```python
from build123d import *

# Parameters (mm, degrees)
FACE001_W        = 15
FACE001_H        = 12
EXTRUDE001_DEPTH = 8
FILLET001_R      = 1
SKETCH_W         = 15
SKETCH_H         = 12
EXTRUDE_DEPTH    = 32
FILLET_R         = 1


with BuildPart() as fillet001:
    # Face001 → Extrude001 (new body)
    with BuildSketch(Plane(origin=(7.5, -32, 6), x_dir=(1, 0, 0), z_dir=(0, 1, 0))):
        Rectangle(FACE001_W, FACE001_H)
    extrude(amount=EXTRUDE001_DEPTH)


with BuildPart() as fillet001_1:
    # Extrude001 placement: moved
    add(fillet001.part.moved(Location((0, -8, 0))))

    # Fillet001
    fillet001_edges = [fillet001_1.edges().sort_by_distance(p)[0] for p in [
        (15, -36, 12),
        (0, -36, 12),
        (7.5, -40, 12),
        (0, -36, 0),
        (0, -40, 6),
        (15, -36, 0),
        (7.5, -40, 0),
        (15, -40, 6),
    ]]
    fillet(fillet001_edges, radius=FILLET001_R)


with BuildPart() as fusion:
    # Sketch → Extrude (new body)
    with BuildSketch(Plane.XZ):
        with Locations((7.5, 6)):
            Rectangle(SKETCH_W, SKETCH_H)
        Polygon((1.775, 10), (13.225, 10), (13.225, 3.8), (11.5, 3.8), (11.5, 2.75), (3.5, 2.75), (3.5, 3.8), (1.775, 3.8), align=None, mode=Mode.SUBTRACT)
    extrude(amount=EXTRUDE_DEPTH)

    # Fillet
    fillet_edges = [fusion.edges().sort_by_distance(p)[0] for p in [
        (0, -16, 0),
        (15, -16, 0),
        (15, -16, 12),
        (0, -16, 12),
    ]]
    fillet(fillet_edges, radius=FILLET_R)

    # Fusion: union Fillet001
    add(fillet001_1.part)


solid = fusion.part
```
Source: CAD feature listing. Evaluate the final solid. Frame: model axes, mm. A direction names the side the tool comes from. Give positions to 0.01 mm unless a question says otherwise; leave off trailing zeros. Write each loop counter-clockwise with the first axis right and the second up, starting at its lowest first coordinate (ties: lowest second). Pieces come first, ordered by that corner, then holes.
1. Section query A-A (y = -7). Return the cut outline in (x, z) (3 decimals), then the cut area to 3 significant figures.
2. Pull-direction query (X, two-part tool) for faces 3 (the face through (0.285, -39.699, 5.93)), 4 (the face through (7.591, -39.699, 0.285)), 5 (the face through (7, -16, 10)); classes: +X half, -X half, draft (parallel to the pull), parting line (faces both ways), or undercut.
3. Material intervals for line 1 along X through (y, z) = (-10, 4.25) (3 decimals); line 2 along Z through (x, y) = (6.5, -15.5); line 3 along Z through (x, y) = (12, -23), sorted ascending.
4. Access query for faces 1 (the face through (0, -20, 6)), 2 (the face through (12, -16, 3.8)). Directions: +Z, -Z, +X, -X, +Y, -Y. A direction counts if a zero-diameter tool reaches every point of the face in a straight line with its end or side. Return the directions, or none.
5. Section query B-B (z = 7.75). Return the cut outline in (x, y) (3 decimals).
6. First-contact query: pin 1 (2 mm diameter, centred on x = 6.5, z = 6, fed in from +Y). Flat tip, straight axial feed; report the tip coordinate or a pass-through.
7. Section query C-C (x = 5.25). Return the cut outline in (y, z), then the cut area to 3 significant figures.
Output values:
1. outline: (0, 1) arc R1 ccw to (1, 0) - (14, 0) arc R1 ccw to (15, 1) - (15, 11) arc R1 ccw to (14, 12) - (1, 12) arc R1 ccw to (0, 11) - close; hole (1.775, 3.8) - (3.5, 3.8) - (3.5, 2.75) - (11.5, 2.75) - (11.5, 3.8) - (13.225, 3.8) - (13.225, 10) - (1.775, 10) - close
1. area: 99.8 mm2
2. face 3: -X half
2. face 4: draft
2. face 5: undercut
3. line 1: x = 0 to 1.775, 13.225 to 15
3. line 2: z = 0 to 2.75, 10 to 12
3. line 3: z = 0 to 3.8, 10 to 12
4. face 1: +Z, -Z, -X, +Y, -Y
4. face 2: +Y
5. outline: (0, -39) arc R1 ccw to (1, -40) - (14, -40) arc R1 ccw to (15, -39) - (15, 0) - (13.225, 0) - (13.225, -32) - (1.775, -32) - (1.775, 0) - (0, 0) - close
6. pin 1: stops at y = -32
7. outline: (-40, 1) arc R1 ccw to (-39, 0) - (0, 0) - (0, 2.75) - (-32, 2.75) - (-32, 10) - (0, 10) - (0, 12) - (-39, 12) arc R1 ccw to (-40, 11) - close
7. area: 248 mm2
